For this review, take the finished solid that the model builds, in its own axes (mm). A direction names the side the tool comes from. Give positions to 0.01 mm unless a question says otherwise; leave off trailing zeros. Loops run counter-clockwise (first coordinate to the right, second up) from the corner with the lowest first, then second, coordinate; pieces in that order, holes last.
```python
from build123d import *

# Parameters (mm, degrees)
SKETCH_1_W          = 170
SKETCH_1_H          = 180
EXTRUDE_1_DEPTH     = 30
CHAMFER_1_SIZE      = 50
SKETCH_3_R          = 76
CUT_EXTRUDE_1_DEPTH = 10
SKETCH_4_R          = 30
CUT_EXTRUDE_2_DEPTH = 126.39936204
SKETCH_5_W          = 40
SKETCH_5_H          = 15
CUT_EXTRUDE_3_DEPTH = 10


with BuildPart() as part:
    # 草图1 → 凸台-拉伸1 (new body)
    with BuildSketch(Plane(origin=(0, 0, 0), x_dir=(1, 0, 0), z_dir=(0, 1, 0))):
        Rectangle(SKETCH_1_W, SKETCH_1_H)
    extrude(amount=EXTRUDE_1_DEPTH)

    # 倒角1
    chamfer_1_edges = [part.edges().sort_by_distance(p)[0] for p in [
        (-85, 15, -90),
        (85, 15, -90),
    ]]
    chamfer(chamfer_1_edges, length=CHAMFER_1_SIZE)

    # 草图3 → 切除-拉伸1 (cut)
    with BuildSketch(Plane(origin=(0, 30, 0), x_dir=(1, 0, 0), z_dir=(0, 1, 0))):
        with Locations(Location((0, 0, 0), (0, 0, 270))):
            Circle(SKETCH_3_R)
    extrude(amount=-CUT_EXTRUDE_1_DEPTH, mode=Mode.SUBTRACT)

    # 草图4 → 切除-拉伸2 (cut, through all)
    with BuildSketch(Plane(origin=(0, 20, 0), x_dir=(1, 0, 0), z_dir=(0, 1, 0))):
        with Locations(Location((0, 0, 0), (0, 0, 270))):
            Circle(SKETCH_4_R)
    extrude(amount=-CUT_EXTRUDE_2_DEPTH, mode=Mode.SUBTRACT)

    # 草图5 → 切除-拉伸3 (cut)
    with BuildSketch(Plane(origin=(0, 0, -90), x_dir=(-1, 0, 0), z_dir=(0, 0, -1))):
        with Locations((0, 12.5)):
            Rectangle(SKETCH_5_W, SKETCH_5_H)
    extrude(amount=-CUT_EXTRUDE_3_DEPTH, mode=Mode.SUBTRACT)


solid = part.part
```
Q1. For pin 1 Ø3 at (x, z) = (4, -85) entering from -Y; pin 2 Ø7.5 at (x, y) = (-2.5, 14.5) entering from -Z; pin 3 Ø8 at (y, z) = (12.5, -86.5) entering from +X; pin 4 Ø3 at (x, y) = (44.5, 15) entering from -Z, all flat-tipped, find the tip position at first contact; note any pin that passes through.
Answers:
pin 1: stops at y = 0
pin 2: stops at z = -80
pin 3: stops at x = 42.5
pin 4: stops at z = -82
Q2. For probe 1 along Z at (x, y) = (-0.5, 20.5); probe 2 along X at (y, z) = (15.5, 0); probe 3 along X at (y, z) = (22, 0), list the stretches that pass through material, from the lowest coordinate up.
Answers:
probe 1: z = -90 to -76, 76 to 90
probe 2: x = -85 to -30, 30 to 85
probe 3: x = -85 to -76, 76 to 85
Q3. Consider section C-C on y = 25. Give the boundary of the cut face in (x, z), plus the area to 3 significant figures.
Answers:
outline: (-85, -40) - (-35, -90) - (35, -90) - (85, -40) - (85, 90) - (-85, 90) - close; hole circle Ø152 at (0, 0)
area: 9,950 mm2
Q4. Consider section B-B on z = 0. Give the boundary of the cut face in (x, y).
Answers:
outline: (-85, 0) - (-30, 0) - (-30, 20) - (-76, 20) - (-76, 30) - (-85, 30) - close; (30, 0) - (85, 0) - (85, 30) - (76, 30) - (76, 20) - (30, 20) - close
Q5. Consider section D-D on z = -72. Give the boundary of the cut face in (x, y).
Answers:
outline: (-53, 0) - (53, 0) - (53, 30) - (24.33, 30) - (24.33, 20) - (-24.33, 20) - (-24.33, 30) - (-53, 30) - close
Q6. Mouldability with a two-part tool opening along Z and no side actions: class faces 1 (the cylindrical face through (1.32, 10.14, -29.97)), 2 (the flat face through (0, 5, -85)), 3 (the flat face through (-60, 15, -65)) as +Z half, -Z half, draft (parallel to the pull), parting line (faces both ways), or undercut.
Answers:
face 1: undercut
face 2: draft
face 3: -Z half
Q7. Machinability: for faces 4 (the flat face through (85, 15, 26)), 5 (the flat face through (1, 20, 33)), 6 (the flat face through (0, 20, -85)), which of the approach directions +Z, -Z, +X, -X, +Y, -Y give a long, thin tool a straight path to every point of the face, cutting with its end or side? Answer none if there is none.
Answers:
face 4: +Z, -Z, +X, +Y, -Y
face 5: +Y
face 6: -Z
Q8. Consider section A-A on x = 0. Give the boundary of the cut face in (y, z), plus the area to 3 significant figures.
Answers:
outline: (0, -90) - (5, -90) - (5, -80) - (20, -80) - (20, -90) - (30, -90) - (30, -76) - (20, -76) - (20, -30) - (0, -30) - close; (0, 30) - (20, 30) - (20, 76) - (30, 76) - (30, 90) - (0, 90) - close
area: 2,530 mm2
